from build123d import *

# Parameters (mm, degrees)
F0_W     = 90
F0_H     = 50
F1_DEPTH = 11.7
F3_R     = 3.5
F4_DEPTH = 8.2
F7_DEPTH = 6.2
F8_R     = 5


with BuildPart() as f1:
    # F0 (on Top) → F1 (new body)
    with BuildSketch(Plane.XY):
        Rectangle(F0_W, F0_H)
    extrude(amount=F1_DEPTH)

    # F3 (on face) → F4 (cut)
    with BuildSketch(Plane.XY.offset(11.7)):
        with Locations((19.886918, 0)):
            Circle(F3_R)
    extrude(amount=-F4_DEPTH, mode=Mode.SUBTRACT)

    # F6 (on offset) → F7 (cut)
    with BuildSketch(Plane.XY.offset(3.5)):
        Polygon((24.876553, 4.19079), (18.762908, 6.398354), (13.794278, 2.207565), (14.939294, -4.19079), (21.052939, -6.398354), (26.021569, -2.207565), align=None)
    extrude(amount=F7_DEPTH, mode=Mode.SUBTRACT)

    # F8
    f8_edges = [f1.edges().sort_by_distance(p)[0] for p in [
        (0, -25, 11.7),
        (45, 0, 11.7),
        (0, 25, 11.7),
        (45, -25, 5.85),
        (45, 25, 5.85),
    ]]
    fillet(f8_edges, radius=F8_R)


solid = f1.part
Input: part model. Units: mm. Frame: model coordinates. A direction names the side the tool comes from. Give positions to 0.01 mm unless a question says otherwise; leave off trailing zeros. Order: outer loops, then holes, each group sorted by start corner. A loop starts at its lowest first (then second) coordinate and runs counter-clockwise, first axis right, second up. Notation, with made-up numbers: M 57,70.25 L 98,70.25 A10 cw 98,76.25 Z; hole C -7,23 d4. An arc over 180 degrees is marked long. Answer as a JSON object with one key per item and string values.
1. Reachability of faces 1 (the cylindrical face through (43, -24, 3)), 2 (the flat face through (25.457, 0.947, 6.557)) from +Z, -Z, +X, -X, +Y, -Y: full face, straight path, thin tool, end or side. Return the list, or none.
Result sheet:
{"face 1": "+Z, -Z, +X, -Y", "face 2": "none"}
2. Cut plane C-C, the plane x = 20. Output: boundary loops of the cut face in (y, z), and give its area (3 significant figures).
Result sheet:
{"outline": "M -25,0 L 25,0 L 25,6.7 A5 ccw 20,11.7 L 3.5,11.7 L 3.5,9.7 L 5.95,9.7 L 5.95,3.5 L -6.02,3.5 L -6.02,9.7 L -3.5,9.7 L -3.5,11.7 L -20,11.7 A5 ccw -25,6.7 Z", "area": "486 mm²"}
3. Cut plane B-B, the plane y = 0. Output: boundary loops of the cut face in (x, z).
Result sheet:
{"outline": "M -45,0 L 45,0 L 45,6.7 A5 ccw 40,11.7 L 23.39,11.7 L 23.39,9.7 L 25.63,9.7 L 25.63,3.5 L 14.19,3.5 L 14.19,9.7 L 16.39,9.7 L 16.39,11.7 L -45,11.7 Z"}
4. Ray query, line 1 (X direction, y = -1, z = 10.75); line 2 (Y direction, x = -33, z = 10.75); line 3 (X direction, y = -17.5, z = 8). Return the intervals inside material, ascending. Write a range as [from, to].
Result sheet:
{"line 1": "[-45, 16.53], [23.24, 42.93]", "line 2": "[-22.93, 22.93]", "line 3": "[-45, 44.83]"}
5. Pull-direction query (X, two-part tool) for faces 3 (the flat face through (-3, -25, 3)), 4 (the cylindrical face through (43, 24, 3)), 5 (the cylindrical face through (23.225, 1.051, 10.714)), 6 (the flat face through (-45, 0, 6)); classes: +X half, -X half, draft (parallel to the pull), parting line (faces both ways), or undercut.
Result sheet:
{"face 3": "draft", "face 4": "+X half", "face 5": "undercut", "face 6": "-X half"}
6. First-contact query: P1, Ø11, axis at x = 19.89, y = 0, coming from the -Z side. Flat tip, straight axial feed; report the tip coordinate or a pass-through.
Result sheet:
{"P1": "z = 0"}
7. Cut plane A-A, the plane x = 0.5. Output: boundary loops of the cut face in (y, z).
Result sheet:
{"outline": "M -25,0 L 25,0 L 25,6.7 A5 ccw 20,11.7 L -20,11.7 A5 ccw -25,6.7 Z"}
